The model under review builds one solid part; all positions refer to its coordinate system, in mm. A direction names the side the tool comes from. Coordinates: 2 decimals unless noted, no trailing zeros. Loops run counter-clockwise (first coordinate to the right, second up) from the corner with the lowest first, then second, coordinate; pieces in that order, holes last. Notation, with made-up numbers: M 11.25,3 L 32.25,3 A23 ccw 32.25,41 Z; hole C 77.5,-20.5 d9. An arc over 180 degrees is marked long. Use one line per item in the form item = value.
```python
from build123d import *

# Parameters (mm, degrees)
SKETCH_2_W           = 100
SKETCH_2_H           = 40
EXTRUDE_1_DEPTH      = 150
SKETCH_3_W           = 90
SKETCH_3_H           = 32
CUT_EXTRUDE_1_DEPTH  = 145
SKETCH_4_W           = 30
SKETCH_4_H           = 115
CUT_EXTRUDE_2_DEPTH  = 20
SKETCH_5_W           = 35
SKETCH_5_H           = 115
CUT_EXTRUDE_3_DEPTH  = 20
SKETCH_6_W           = 120
SKETCH_6_H           = 31
CUT_EXTRUDE_4_DEPTH  = 207
SKETCH_7_R           = 1.5
CUT_EXTRUDE_5_DEPTH  = 15
SKETCH_8_R           = 2.5
CUT_EXTRUDE_6_DEPTH  = 15
SKETCH_11_W          = 100
SKETCH_11_H          = 150
CUT_EXTRUDE_7_DEPTH  = 20
SKETCH_12_R          = 1.6
EXTRUDE_3_DEPTH      = 6
SKETCH_13_W          = 4.955411511
SKETCH_13_H          = 10
SKETCH_13_W_2        = 5.044588489
EXTRUDE_4_DEPTH      = 10
SKETCH_15_R          = 1.6
CUT_EXTRUDE_8_DEPTH  = 10
SKETCH_16_R          = 1.5
SKETCH_16_R_2        = 2.5
CUT_EXTRUDE_9_DEPTH  = 10
SKETCH_17_R          = 1.5
CUT_EXTRUDE_10_DEPTH = 10
SKETCH_18_R          = 1.5
CUT_EXTRUDE_11_DEPTH = 10
SKETCH_19_R          = 2.5
CUT_EXTRUDE_12_DEPTH = 1
SKETCH_20_R          = 2.5
CUT_EXTRUDE_13_DEPTH = 1


with BuildPart() as part:
    # 草图2 → 凸台-拉伸1 (new body)
    with BuildSketch(Plane.XY):
        Rectangle(SKETCH_2_W, SKETCH_2_H)
    extrude(amount=EXTRUDE_1_DEPTH)

    # 草图3 → 切除-拉伸1 (cut)
    with BuildSketch(Plane.XY.offset(150)):
        with Locations((0.044588489, 1)):
            Rectangle(SKETCH_3_W, SKETCH_3_H)
    extrude(amount=-CUT_EXTRUDE_1_DEPTH, mode=Mode.SUBTRACT)

    # 草图4 → 切除-拉伸2 (cut)
    with BuildSketch(Plane.XZ.offset(20)):
        with Locations((-25, 77.5)):
            Rectangle(SKETCH_4_W, SKETCH_4_H)
        with Locations((25, 77.5)):
            Rectangle(SKETCH_4_W, SKETCH_4_H)
    extrude(amount=-CUT_EXTRUDE_2_DEPTH, mode=Mode.SUBTRACT)

    # 草图5 → 切除-拉伸3 (cut)
    with BuildSketch(Plane(origin=(0, 20, 0), x_dir=(1, 0, 0), z_dir=(0, 1, 0))):
        with Locations((-22.5, -77.5)):
            Rectangle(SKETCH_5_W, SKETCH_5_H)
        with Locations((22.5, -77.5)):
            Rectangle(SKETCH_5_W, SKETCH_5_H)
    extrude(amount=-CUT_EXTRUDE_3_DEPTH, mode=Mode.SUBTRACT)

    # 草图6 → 切除-拉伸4 (cut)
    with BuildSketch(Plane.ZY.offset(50)):
        with Locations((75, 0.5)):
            Rectangle(SKETCH_6_W, SKETCH_6_H)
    extrude(amount=-CUT_EXTRUDE_4_DEPTH, mode=Mode.SUBTRACT)

    # 草图7 → 切除-拉伸5 (cut)
    with BuildSketch(Plane.XZ.offset(20)):
        with Locations(Location((-5, 134, 0), (0, 0, 270))):
            Circle(SKETCH_7_R)
        with Locations(Location((5, 134, 0), (0, 0, 270))):
            Circle(SKETCH_7_R)
        with Locations(Location((5, 124, 0), (0, 0, 270))):
            Circle(SKETCH_7_R)
        with Locations(Location((-5, 124, 0), (0, 0, 270))):
            Circle(SKETCH_7_R)
    extrude(amount=-CUT_EXTRUDE_5_DEPTH, mode=Mode.SUBTRACT)

    # 草图8 → 切除-拉伸6 (cut)
    with BuildSketch(Plane.XZ.offset(20)):
        with Locations(Location((0, 129, 0), (0, 0, 270))):
            Circle(SKETCH_8_R)
    extrude(amount=-CUT_EXTRUDE_6_DEPTH, mode=Mode.SUBTRACT)

    # 草图11 → 切除-拉伸7 (cut)
    with BuildSketch(Plane(origin=(0, 20, 0), x_dir=(1, 0, 0), z_dir=(0, 1, 0))):
        with Locations((0, -75)):
            Rectangle(SKETCH_11_W, SKETCH_11_H)
    extrude(amount=-CUT_EXTRUDE_7_DEPTH, mode=Mode.SUBTRACT)

    # 草图12 → 凸台-拉伸3 (add)
    # profile 1 of 4: a face of its own
    with BuildSketch(Plane(origin=(0, 0, 0), x_dir=(1, 0, 0), z_dir=(0, 1, 0))):
        with BuildLine():
            Line((-50, 0), (-60, 0))
            ThreePointArc((-60, 0), (-65, -5), (-60, -10))
            Line((-60, -10), (-50, -10))
            Line((-50, -10), (-50, 0))
        make_face()
        with Locations(Location((-60, -5, 0), (0, 0, 270))):
            Circle(SKETCH_12_R, mode=Mode.SUBTRACT)
    # profile 2 of 4: a face of its own
    with BuildSketch(Plane(origin=(0, 0, 0), x_dir=(1, 0, 0), z_dir=(0, 1, 0))):
        with BuildLine():
            Line((50, 0), (50, -10))
            Line((50, -10), (60, -10))
            ThreePointArc((60, -10), (65, -5), (60, 0))
            Line((60, 0), (50, 0))
        make_face()
        with Locations(Location((60, -5, 0), (0, 0, 270))):
            Circle(SKETCH_12_R, mode=Mode.SUBTRACT)
    # profile 3 of 4: a face of its own
    with BuildSketch(Plane(origin=(0, 0, 0), x_dir=(1, 0, 0), z_dir=(0, 1, 0))):
        with BuildLine():
            Line((45.044588489, -125), (45.044588489, -135))
            Line((45.044588489, -135), (55.044588489, -135))
            ThreePointArc((55.044588489, -135), (60.044588489, -130), (55.044588489, -125))
            Line((55.044588489, -125), (45.044588489, -125))
        make_face()
        with Locations(Location((55.044588489, -130, 0), (0, 0, 270))):
            Circle(SKETCH_12_R, mode=Mode.SUBTRACT)
    # profile 4 of 4: a face of its own
    with BuildSketch(Plane(origin=(0, 0, 0), x_dir=(1, 0, 0), z_dir=(0, 1, 0))):
        with BuildLine():
            Line((-44.955411511, -125), (-44.955411511, -135))
            Line((-44.955411511, -135), (-54.955411511, -135))
            ThreePointArc((-54.955411511, -135), (-59.955411511, -130), (-54.955411511, -125))
            Line((-54.955411511, -125), (-44.955411511, -125))
        make_face()
        with Locations(Location((-54.955411511, -130, 0), (0, 0, 270))):
            Circle(SKETCH_12_R, mode=Mode.SUBTRACT)
    extrude(amount=-EXTRUDE_3_DEPTH)

    # 草图13 → 凸台-拉伸4 (add)
    with BuildSketch(Plane.XZ.offset(6)):
        with Locations((47.522294245, 130)):
            Rectangle(SKETCH_13_W, SKETCH_13_H)
        with Locations((-47.477705755, 130)):
            Rectangle(SKETCH_13_W_2, SKETCH_13_H)
    extrude(amount=EXTRUDE_4_DEPTH)

    # 草图15 → 切除-拉伸8 (cut)
    with BuildSketch(Plane.XZ.offset(20)):
        with Locations(Location((0, 144.5, 0), (0, 0, 270))):
            Circle(SKETCH_15_R)
    extrude(amount=-CUT_EXTRUDE_8_DEPTH, mode=Mode.SUBTRACT)

    # 草图16 → 切除-拉伸9 (cut)
    with BuildSketch(Plane(origin=(0, -15, 0), x_dir=(1, 0, 0), z_dir=(0, 1, 0))):
        with Locations(Location((0, -74, 0), (0, 0, 270))):
            Circle(SKETCH_16_R)
        with Locations(Location((0, -19, 0), (0, 0, 270))):
            Circle(SKETCH_16_R_2)
        with Locations(Location((-5, -14, 0), (0, 0, 270))):
            Circle(SKETCH_16_R)
        with Locations(Location((5, -14, 0), (0, 0, 270))):
            Circle(SKETCH_16_R)
        with Locations(Location((-5, -24, 0), (0, 0, 270))):
            Circle(SKETCH_16_R)
        with Locations(Location((5, -24, 0), (0, 0, 270))):
            Circle(SKETCH_16_R)
        with Locations(Location((-5, -69, 0), (0, 0, 270))):
            Circle(SKETCH_16_R)
        with Locations(Location((5, -69, 0), (0, 0, 270))):
            Circle(SKETCH_16_R)
        with Locations(Location((5, -79, 0), (0, 0, 270))):
            Circle(SKETCH_16_R)
        with Locations(Location((-5, -79, 0), (0, 0, 270))):
            Circle(SKETCH_16_R)
    extrude(amount=-CUT_EXTRUDE_9_DEPTH, mode=Mode.SUBTRACT)

    # 草图17 → 切除-拉伸10 (cut)
    with BuildSketch(Plane.XZ.offset(20)):
        with Locations(Location((-45, 74, 0), (0, 0, 270))):
            Circle(SKETCH_17_R)
        with Locations(Location((-45, 54, 0), (0, 0, 270))):
            Circle(SKETCH_17_R)
        with Locations(Location((45, 54, 0), (0, 0, 270))):
            Circle(SKETCH_17_R)
        with Locations(Location((45, 74, 0), (0, 0, 270))):
            Circle(SKETCH_17_R)
    extrude(amount=-CUT_EXTRUDE_10_DEPTH, mode=Mode.SUBTRACT)

    # 草图18 → 切除-拉伸11 (cut)
    with BuildSketch(Plane.XY.offset(5)):
        with Locations((-7.089720892, -2.5)):
            Circle(SKETCH_18_R)
        with Locations((2.910279108, -2.5)):
            Circle(SKETCH_18_R)
        with Locations((-7.089720892, -12.5)):
            Circle(SKETCH_18_R)
        with Locations((2.910279108, -12.5)):
            Circle(SKETCH_18_R)
    extrude(amount=-CUT_EXTRUDE_11_DEPTH, mode=Mode.SUBTRACT)

    # 草图19 → 切除-拉伸12 (cut)
    with BuildSketch(Plane(origin=(0, -15, 0), x_dir=(1, 0, 0), z_dir=(0, 1, 0))):
        with Locations(Location((5, -79, 0), (0, 0, 270))):
            Circle(SKETCH_19_R)
        with Locations(Location((-5, -79, 0), (0, 0, 270))):
            Circle(SKETCH_19_R)
        with Locations(Location((-5, -69, 0), (0, 0, 270))):
            Circle(SKETCH_19_R)
        with Locations(Location((5, -69, 0), (0, 0, 270))):
            Circle(SKETCH_19_R)
    extrude(amount=-CUT_EXTRUDE_12_DEPTH, mode=Mode.SUBTRACT)

    # 草图20 → 切除-拉伸13 (cut)
    with BuildSketch(Plane(origin=(0, -15, 0), x_dir=(1, 0, 0), z_dir=(0, 1, 0))):
        with Locations(Location((0, -74, 0), (0, 0, 270))):
            Circle(SKETCH_20_R)
    extrude(amount=-CUT_EXTRUDE_13_DEPTH, mode=Mode.SUBTRACT)


solid = part.part
```
1. Add section B-B (x = -21). State the section outline as (y, z) points, then the cut area to 3 significant figures.
Response values:
outline = M -20,0 L 0,0 L 0,5 L -15,5 L -15,20 L -20,20 Z; M -20,135 L -15,135 L -15,150 L -20,150 Z
area = 250 mm^2
2. The part is to be moulded in two halves that separate along Y. For faces 6 (the face through (-1, 0, 2)), 7 (the face through (-8.59, -12.43, 2.54)), 8 (the face through (5.07, -17.46, 12.5)), say which applies: pulls with the +Y half, pulls with the -Y half, needs draft (parallel to the pull), parting line crosses it, or undercut.
Response values:
face_6 = pulls with the +Y half
face_7 = undercut
face_8 = needs draft
3. Add section C-C (z = 144.5). State the section outline as (x, y) points.
Response values:
outline = M -50,-20 L -1.6,-20 L -1.6,-15 L -44.96,-15 L -44.96,0 L -50,0 Z; M 1.6,-20 L 50,-20 L 50,0 L 45.04,0 L 45.04,-15 L 1.6,-15 Z
4. Machinability: for faces 1 (the face through (25, -18, 135)), 2 (the face through (52, -3, 135)), 3 (the face through (-55, -3, 10)), 4 (the face through (-2, -16, 74)), 5 (the face through (-48, -8, 15)), which of the approach directions +Z, -Z, +X, -X, +Y, -Y give a long, thin tool a straight path to every point of the face, cutting with its end or side? Answer none if there is none.
Response values:
face_1 = +Y, -Y
face_2 = +Z, +X, +Y, -Y
face_3 = -X, +Y, -Y
face_4 = +Y
face_5 = +X, -X, +Y
5. Wall thickness on line 1 along X through (y, z) = (-15.7, 74); line 2 along X through (y, z) = (-4.65, 130); line 3 along X through (y, z) = (-15.95, 124): over which ranges is each line inside the solid? List them lowest first. Write a range as from..to.
Response values:
line_1 = -50..-46.5, -43.5..-40, -10..-2.5, 2.5..10, 40..43.5, 46.5..50
line_2 = -59.96..-56.56, -53.36..-44.96, 45.04..53.44, 56.64..60.04
line_3 = -50..-40, -10..-6.5, -3.5..3.5, 6.5..10, 40..50
6. Insertion check: P1, Ø8, axis at x = 44.5, z = 107.5, coming from the +Y side; P2, Ø10, axis at y = -7, z = 21.5, coming from the +X side; P3, Ø6.5, axis at x = 0, z = 74, coming from the -Y side. Each pin has a flat end and moves straight along its axis. Give the tip position at first contact, or say it passes through.
Response values:
P1 = -15
P2 = through
P3 = -20
7. Add section A-A (z = 117). State the section outline as (x, y) points.
Response values:
outline = M -50,-20 L -40,-20 L -40,-15 L -50,-15 Z; M -10,-20 L 10,-20 L 10,-15 L -10,-15 Z; M 40,-20 L 50,-20 L 50,-15 L 40,-15 Z
